Geometry: see drawing. Coordinates: mm, zero at the bounding-box minimum. Coordinates: 2 decimals unless noted, no trailing zeros. Order: outer loops, then holes, each group sorted by start corner. A loop starts at its lowest first (then second) coordinate and runs counter-clockwise, first axis right, second up. Notation, with made-up numbers: (24.5, 41) - (53.5, 41) arc R24 cw to (53.5, 69) - close; hole circle Ø1 at (70.25, 40). An arc over 180 degrees is marked (long way). Use a Markdown table: item, result. Add a question column.
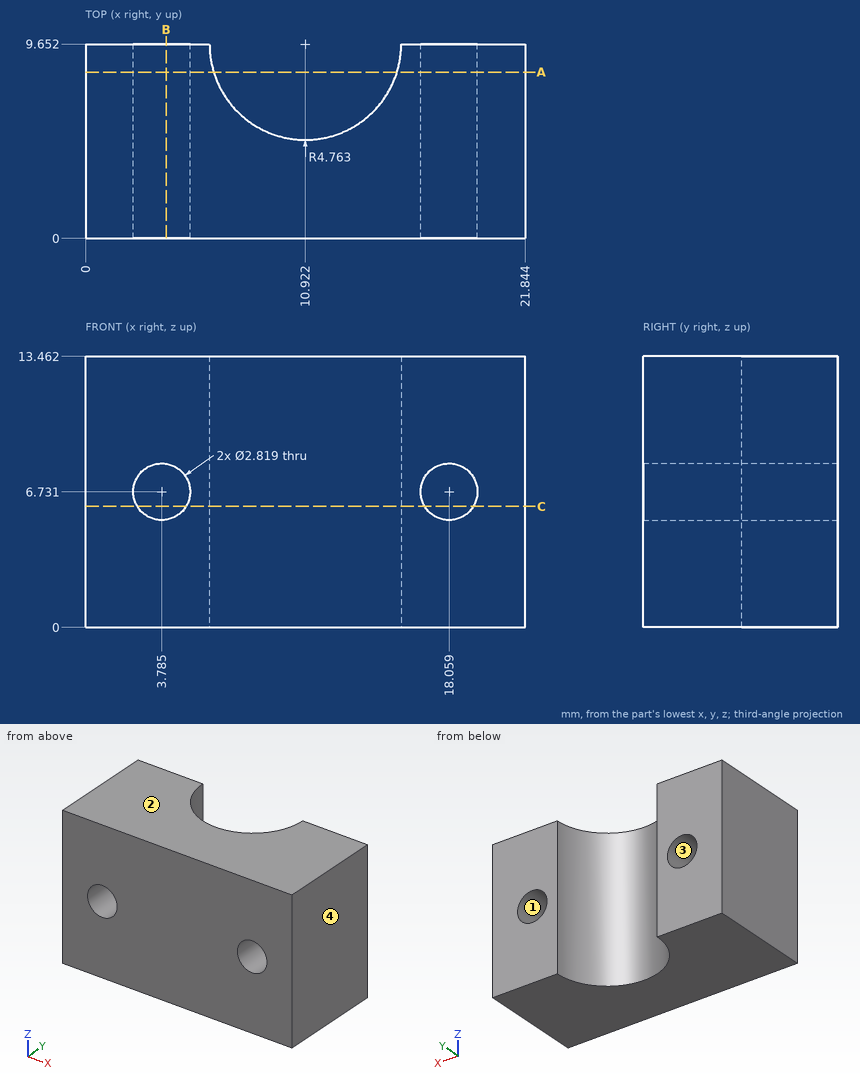
1) Cut plane B-B (x = 4). Return the cut outline in (y, z) (1 decimal), and give its area (3 significant figures).
2) Cut plane C-C (z = 6). Return the cut outline in (x, y) (1 decimal).
3) Pull-direction query (X, two-part tool) for the marked faces 1, 2, 3 and 4; classes: pulls with the +X half, pulls with the -X half, needs draft (parallel to the pull), parting line crosses it, or undercut.
4) Cut plane A-A (y = 8.25). State how many separate pieces and enclosed holes the cut face has, and give its area (3 significant figures).
5) Material intervals for L1, parallel to X at y = 6.75, z = 7 (1 decimal); L2, parallel to Z at x = 18, y = 4; L3, parallel to X at y = 6.25, z = 5.25 (1 decimal), sorted ascending.
Computed:
| question | item | result |
|---|---|---|
| 1 | outline | (0, 0) - (9.7, 0) - (9.7, 5.3) - (0, 5.3) - close; (0, 8.1) - (9.7, 8.1) - (9.7, 13.5) - (0, 13.5) - close |
| 1 | area | 103 mm2 |
| 2 | outline | (0, 0) - (2.6, 0) - (2.6, 9.7) - (0, 9.7) - close; (5, 0) - (16.9, 0) - (16.9, 9.7) - (15.7, 9.7) arc R4.8 cw to (6.2, 9.7) - (5, 9.7) - close; (19.3, 0) - (21.8, 0) - (21.8, 9.7) - (19.3, 9.7) - close |
| 3 | face 1 | undercut |
| 3 | face 2 | needs draft |
| 3 | face 3 | undercut |
| 3 | face 4 | pulls with the +X half |
| 4 | separate pieces | 2 |
| 4 | enclosed holes | 2 |
| 4 | area | 159 mm2 |
| 5 | L1 | x = 0 to 2.4, 5.2 to 7.1, 14.7 to 16.7, 19.4 to 21.8 |
| 5 | L2 | z = 0 to 5.32, 8.14 to 13.46 |
| 5 | L3 | x = 0 to 7.6, 14.3 to 21.8 |
